CAD build for the part. Positions are in the model's coordinates, mm. A direction names the side the tool comes from. Give positions to 0.01 mm unless a question says otherwise; leave off trailing zeros. Loops run counter-clockwise (first coordinate to the right, second up) from the corner with the lowest first, then second, coordinate; pieces in that order, holes last.
Item 1: Saw through at A-A on x = 10.75. Give the cut face in (y, z).
Item 2: Mould opens along Y. For faces 4 (the cylindrical face through (0.299, 2.642, 0.832)), 5 (the flat face through (16, 0, 0)), 6 (the flat face through (0.68, -0.51, -0.86)) say: released by +Y, released by -Y, zero draft, split by the parting line, or undercut.
Item 3: Which spindle directions (+Z, -Z, +X, -X, +Y, -Y) get a long thin tool onto all of the face, cutting with end or side? Do faces 1 (the flat face through (1, -1, 0)), 2 (the cylindrical face through (8.68, -1.5, -0.07)), 3 (the flat face through (0, -1.2, 0)). Say none if no direction does.
Item 4: Drop flat-ended pins along their axis: P1, Ø3, axis at x = 5, y = -2, coming from the -Z side; P2, Ø3, axis at x = 8.5, z = -2, coming from the +Y side; P3, Ø1.5, axis at x = 8, y = 1.5, coming from the +Z side. Give the stop position or say it passes through.
Item 5: Probe probe 1 along Z at (x, y) = (10, 0); probe 2 along Y at (x, z) = (1, 0.85); probe 3 along Z at (x, y) = (3.5, 0.8). List the from-to ranges inside material, lowest first.
Autodesk Inventor part; units mm, degrees
ref_plane "Work Plane1" through (104.775, 0, 0) normal (0, 0, -1) x (1, 0, 0)
ref_plane "YZ Plane" through (0, 0, 0) normal (1, 0, 0) x (0, 1, 0)
ref_plane "XZ Plane" through (0, 0, 0) normal (0, 1, 0) x (-1, 0, 0)
sketch "Sketch1" plane through (0, 0, 0) normal (0, 0, 1) x (1, 0, 0)
  line L0 (16, 0) -> (16, 1.5)
  line L1 (16, 1.5) -> (4, 1.5)
  line L2 (4, 1.5) -> (3.6933, 1.5)
  line L3 (0, 2.77) -> (0, 1.1547)
  line L4 (0, 1.1547) -> (1.3, 1.1547)
  line L5 (1.3, 1.1547) -> (1.9667, 0)
  line L6 (1.9667, 0) -> (16, 0)
  line L7 (0, 2.77) -> (0.59, 2.77)
  line L8 (0.59, 2.77) -> (1.86, 1.5)
  line L9 (3.6933, 1.5) -> (1.86, 1.5)
  line L10 (4, 1.5) -> (1.86, 1.5) construction
  line L11 (1.86, 1.5) -> (1.86, 1.5)
  line L12 (-3.2, 0) -> (19.2, 0)
  line L13 (0, -0.554) -> (0, 3.324)
  dimension "d0" = 16
  dimension "d1" = 12
  dimension "d2" = 1.3
  dimension "d3" = 3
  dimension "d6" = 1.86
  dimension "d7" = 45
  dimension "d8" = 2.3094
  dimension "d9" = 60
  dimension "d10" = 5.54
  dimension "d11" = 3
  dimension "d12" = 0.3067
revolve "Body" add sketch "Sketch1" angle 360 about axis through (1.9667, 0, 0) along (1, 0, 0) contours L6 L5 L4 L3 L7 L8 L9 L2 L1 L0
sketch "Sketch2" plane through (0, 0, 0) normal (-1, 0, 0) x (0, 0, 1)
  circle A0 centre (0, 0) radius 1.1547
  line L0 (0, -3.878) -> (0, 3.878)
  line L1 (-3.878, 0) -> (3.878, 0)
  line L2 (1.1547, 0) -> (0.5774, -1)
  line L3 (0.5774, -1) -> (-0.5774, -1)
  line L4 (-0.5774, -1) -> (-1.1547, 0)
  line L5 (-1.1547, 0) -> (-0.5774, 1)
  line L6 (-0.5774, 1) -> (0.5774, 1)
  line L7 (0.5774, 1) -> (1.1547, 0)
  point P0 (0, 1.1547)
extrude "Slot" add sketch "Sketch2" against normal up to next contours L7 A0 | A0 L2 | L6 L0 A0 | A0 L0 L3 | L0 L6 A0 | A0 L3 L0 | L4 A0 | A0 L5
thread "Thread"
chamfer "Chamfer1" distance 0.3067 distance2 0.3067 1 edges at (16, -1.5, 0) measured on face at (16, -0.3743, -0.3316)
ref_plane "Work Plane1" through (104.775, 0, 0) normal (0, 0, -1) x (1, 0, 0)
equation "\"d0\" = NLG"
equation "\"d1\" = GEL"
equation "\"d2\" = INTI"
equation "\"d3\" = GD"
equation "\"d6\" = KOH"
equation "\"d7\" = 0.5 * SEWI"
equation "\"d8\" = 1.1547 * SW"
equation "\"d10\" = KOD"
equation "\"d11\" = BDM"
equation "\"d12\" = GAL"
equation "\"d15\" = GEL"
equation "\"d17\" = -0.5 * SPD + 0.5 * GD"
equation "\"d18\" = GUL"
equation "\"NLG\" = 16"
equation "\"INTI\" = 1.3"
equation "\"GEL\" = 12"
equation "\"GAL\" = 0.61345 * PTC"
equation "\"KOH\" = 1.86"
equation "\"KOD\" = 5.54"
equation "\"GUL\" = 0.61345 * PTC"
equation "\"SPD\" = NND - 1.2269 * PTC"
equation "\"BDM\" = NND"
equation "\"GD\" = NND"
equation "\"SEWI\" = 90deg"
equation "\"SW\" = 2"
equation "\"TOA\" = 30deg"
equation "\"GD1\" = THREADDIA - 1.2269 * PTC"
equation "\"EPV\" = 3.36"
equation "\"THREADDIA\" = 3"
equation "\"PTC\" = 0.5"
equation "\"NND\" = 3"
equation "\"E0\" = 2.31"
equation "\"THREADDESC\" = 1.2345"
properties part number "M3 x  16 - Socket Csk Screw (A2)" material "Stainless Steel"
Results below:
1. outline: circle Ø3 at (0, 0)
2. face 4: split by the parting line
2. face 5: zero draft
2. face 6: undercut
3. face 1: -X
3. face 2: +X
3. face 3: +Z, -Z, -X, +Y, -Y
4. P1: stops at z = -1.41
4. P2: stops at y = 1.41
4. P3: stops at z = 1.3
5. probe 1: z = -1.5 to 1.5
5. probe 2: y = -2.2 to -0.53, 0.53 to 2.2
5. probe 3: z = -1.27 to 1.27
